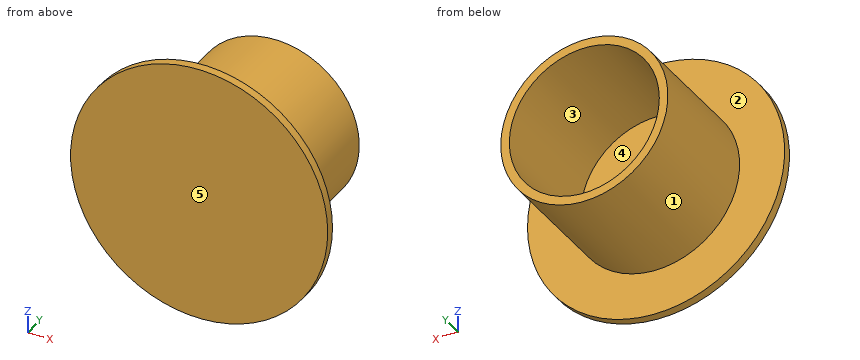
from build123d import *

# Parameters (mm, degrees)
SKETCH1_R           = 19.5
SKETCH1_R_2         = 17.5
BOSS_EXTRUDE1_DEPTH = 30
SKETCH2_R           = 30
BOSS_EXTRUDE2_DEPTH = 2


with BuildPart() as part:
    # Sketch1 → Boss-Extrude1 (new body)
    with BuildSketch(Plane(origin=(0, 0, 0), x_dir=(1, 0, 0), z_dir=(0, 1, 0))):
        Circle(SKETCH1_R)
        Circle(SKETCH1_R_2, mode=Mode.SUBTRACT)
    extrude(amount=BOSS_EXTRUDE1_DEPTH)

    # Sketch2 → Boss-Extrude2 (add)
    with BuildSketch(Plane.XZ):
        Circle(SKETCH2_R)
    extrude(amount=BOSS_EXTRUDE2_DEPTH)


solid = part.part
Model file for the job. Use its own axes, mm. Face numbers are marked on the shaded views. A direction names the side the tool comes from. Coordinates: 2 decimals unless noted, no trailing zeros. Write each loop counter-clockwise with the first axis right and the second up, starting at its lowest first coordinate (ties: lowest second). Pieces come first, ordered by that corner, then holes. Notation, with made-up numbers: (10.25, -4.5) -> (67.25, -4.5) arc R9 cw to (67.25, -0.5) -> close; hole circle Ø9 at (-33, -18.75). An arc over 180 degrees is marked (long way). One line per item, written item: value. Start each with the question number.
1) Probe probe 1 along Z at (x, y) = (0, 13); probe 2 along Y at (x, z) = (-10.5, 12). List the from-to ranges inside material, lowest first.
2) Slice it at B-B on z = 0. Write the cut outline in (x, y).
3) Flat gauge pins, fed straight in: pin 1 Ø10 at (x, y) = (-23, 25.5) entering from -Z; pin 2 Ø5 at (y, z) = (7, 3.5) entering from -X; pin 3 Ø12 at (x, y) = (10, 1.5) entering from +Z. Where does each tip first touch, or does it go through?
4) Slice it at A-A on x = 0. Write the cut outline in (y, z).
5) Slice it at C-C on y = 16. Write the cut outline in (x, z).
6) Pull direction X, two halves, no side cores. Call the marked faces 1, 2 and 3: +X half, -X half, draft (parallel to the pull), parting line (faces both ways), or undercut.
7) Which spindle directions (+Z, -Z, +X, -X, +Y, -Y) get a long thin tool onto all of the face, cutting with end or side? Do the marked faces 4 and 5. Say none if no direction does.
8) Slice it at D-D on x = 18.5. Write the cut outline in (y, z).
Answers follow:
1. probe 1: -19.5 to -17.5, 17.5 to 19.5
1. probe 2: -2 to 0
2. outline: (-30, -2) -> (30, -2) -> (30, 0) -> (19.5, 0) -> (19.5, 30) -> (17.5, 30) -> (17.5, 0) -> (-17.5, 0) -> (-17.5, 30) -> (-19.5, 30) -> (-19.5, 0) -> (-30, 0) -> close
3. pin 1: z = -7.5
3. pin 2: x = -19.47
3. pin 3: z = 29.71
4. outline: (-2, -30) -> (0, -30) -> (0, -19.5) -> (30, -19.5) -> (30, -17.5) -> (0, -17.5) -> (0, 17.5) -> (30, 17.5) -> (30, 19.5) -> (0, 19.5) -> (0, 30) -> (-2, 30) -> close
5. outline: circle Ø39 at (0, 0); hole circle Ø35 at (0, 0)
6. face 1: parting line
6. face 2: draft
6. face 3: undercut
7. face 4: +Y
7. face 5: +Z, -Z, +X, -X, -Y
8. outline: (-2, -23.62) -> (0, -23.62) -> (0, -6.16) -> (30, -6.16) -> (30, 6.16) -> (0, 6.16) -> (0, 23.62) -> (-2, 23.62) -> close
